from build123d import *

# Parameters (mm, degrees)
SKETCH1_W           = 152.4
SKETCH1_H           = 152.4
BOSS_EXTRUDE1_DEPTH = 25.4
SKETCH3_R           = 3.175
CUT_EXTRUDE1_DEPTH  = 130.830173774
SKETCH4_W           = 12.7
SKETCH4_H           = 12.7
CUT_EXTRUDE2_DEPTH  = 130.830173774
SHELL1_T            = -1.27


with BuildPart() as part:
    # Sketch1 → Boss-Extrude1 (new body)
    with BuildSketch(Plane(origin=(0, 0, 0), x_dir=(1, 0, 0), z_dir=(0, 1, 0))):
        with Locations((1.284269663, 24.829213483)):
            Rectangle(SKETCH1_W, SKETCH1_H)
    extrude(amount=BOSS_EXTRUDE1_DEPTH)

    # Sketch3 → Cut-Extrude1 (cut, through all)
    with BuildSketch(Plane(origin=(0, 25.4, 0), x_dir=(1, 0, 0), z_dir=(0, 1, 0))):
        with Locations(Location((-68.565730337, 94.679213483, 0), (0, 0, 270))):
            Circle(SKETCH3_R)
        with Locations(Location((71.134269663, 94.679213483, 0), (0, 0, 270))):
            Circle(SKETCH3_R)
        with Locations(Location((-68.565730337, -45.020786517, 0), (0, 0, 270))):
            Circle(SKETCH3_R)
        with Locations(Location((71.134269663, -45.020786517, 0), (0, 0, 270))):
            Circle(SKETCH3_R)
    extrude(amount=-CUT_EXTRUDE1_DEPTH, mode=Mode.SUBTRACT)

    # Sketch4 → Cut-Extrude2 (cut, through all)
    with BuildSketch(Plane(origin=(0, 25.4, 0), x_dir=(1, 0, 0), z_dir=(0, 1, 0))):
        with Locations((-10.907730337, 54.801213483)):
            Rectangle(SKETCH4_W, SKETCH4_H)
        with Locations((13.476269663, 54.801213483)):
            Rectangle(SKETCH4_W, SKETCH4_H)
        with Locations((-10.907730337, 35.751213483)):
            Rectangle(SKETCH4_W, SKETCH4_H)
        with Locations((13.476269663, 35.751213483)):
            Rectangle(SKETCH4_W, SKETCH4_H)
        with Locations((13.476269663, 16.701213483)):
            Rectangle(SKETCH4_W, SKETCH4_H)
    extrude(amount=-CUT_EXTRUDE2_DEPTH, mode=Mode.SUBTRACT)

    # Shell1
    shell1_openings = [part.faces().sort_by_distance(p)[0] for p in [
        (-10.907730337, 25.4, -35.751213483),
    ]]
    offset(amount=SHELL1_T, openings=shell1_openings, kind=Kind.INTERSECTION)


solid = part.part
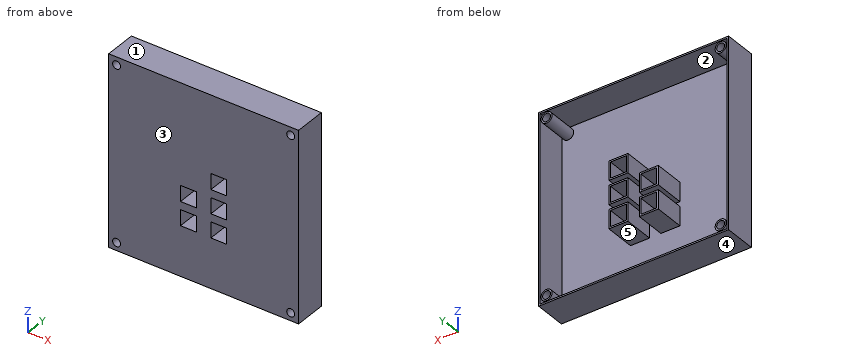
Can you work these out from the model? Positions are in its coordinate system, mm. Face numbers are marked on the shaded views. A direction names the side the tool comes from. Give positions to 0.01 mm unless a question says otherwise; leave off trailing zeros. Write each loop counter-clockwise with the first axis right and the second up, starting at its lowest first coordinate (ties: lowest second). Pieces come first, ordered by that corner, then holes. Notation, with made-up numbers: (12.5, -14.5) -> (38.5, -14.5) arc R11 ccw to (38.5, -3.5) -> close; hole circle Ø5 at (-17.75, 59). An arc over 180 degrees is marked (long way). Answer as a JSON object with one key per item and string values. Group by question number.
Item 1: I'm going to push a flat-ended pin straight in: P1, Ø10, axis at x = -54, z = -77, coming from the +Y side. Where does the tip first touch, or does it pass through?
Item 2: Please list where these lines run through material, in increasing order: line 1 (X direction, y = 15.25, z = -57); line 2 (X direction, y = 5.75, z = 45); line 3 (Z direction, x = -13, y = 4). Write a range as [from, to].
Item 3: For the marked faces 1 and 2, which set-ups out of +Z, -Z, +X, -X, +Y, -Y let a thin tool reach every point of the face, with its end or its side?
Item 4: Suppose I cut it at D-D (z = 6). Please give me the cut outline in (x, y), plus the area to 3 significant figures.
Item 5: Suppose I cut it at C-C (x = 11). State how many separate pieces and enclosed holes the cut face has, plus the area to 3 significant figures.
Item 6: Suppose I cut it at A-A (z = -16.5). Please give me the cut outline in (x, y), plus the area to 3 significant figures.
Item 7: Suppose I cut it at B-B (z = -38). Please give me the cut outline in (x, y).
Item 8: We'd pull the mould along Z, two halves only. Please class the marked faces 3, 4 and 5: +Z half, -Z half, draft (parallel to the pull), parting line (faces both ways), or undercut.
Findings:
{
 "1": {"P1": "stops at y = 1.27"},
 "2": {"line 1": "x = [-74.92, -73.65], [-18.53, -17.26], [-4.56, -3.29], [5.86, 7.13], [19.83, 21.1], [76.21, 77.48]", "line 2": "x = [-74.92, -73.65], [-73.01, -71.74], [-65.39, -64.12], [66.69, 67.96], [74.31, 75.58], [76.21, 77.48]", "line 3": "z = [-101.03, -99.76], [-62.42, -61.15], [-48.45, -47.18], [-43.37, -42.1], [-29.4, -28.13], [50.1, 51.37]"},
 "3": {"face 1": "+Z, +X, -X, +Y, -Y", "face 2": "+Y"},
 "4": {"outline": "(-74.92, 0) -> (77.48, 0) -> (77.48, 25.4) -> (76.21, 25.4) -> (76.21, 1.27) -> (-73.65, 1.27) -> (-73.65, 25.4) -> (-74.92, 25.4) -> close", "area": "255 mm²"},
 "5": {"separate pieces": "4", "enclosed holes": "0", "area": "390 mm²"},
 "6": {"outline": "(-74.92, 0) -> (7.13, 0) -> (7.13, 25.4) -> (5.86, 25.4) -> (5.86, 1.27) -> (-73.65, 1.27) -> (-73.65, 25.4) -> (-74.92, 25.4) -> close; (19.83, 0) -> (77.48, 0) -> (77.48, 25.4) -> (76.21, 25.4) -> (76.21, 1.27) -> (21.1, 1.27) -> (21.1, 25.4) -> (19.83, 25.4) -> close", "area": "300 mm²"},
 "7": {"outline": "(-74.92, 0) -> (-17.26, 0) -> (-17.26, 25.4) -> (-18.53, 25.4) -> (-18.53, 1.27) -> (-73.65, 1.27) -> (-73.65, 25.4) -> (-74.92, 25.4) -> close; (-4.56, 0) -> (7.13, 0) -> (7.13, 25.4) -> (5.86, 25.4) -> (5.86, 1.27) -> (-3.29, 1.27) -> (-3.29, 25.4) -> (-4.56, 25.4) -> close; (19.83, 0) -> (77.48, 0) -> (77.48, 25.4) -> (76.21, 25.4) -> (76.21, 1.27) -> (21.1, 1.27) -> (21.1, 25.4) -> (19.83, 25.4) -> close"},
 "8": {"face 3": "draft", "face 4": "-Z half", "face 5": "undercut"}
}
